Part print with two shaded views. Sizes in mm from the minimum x, y, z corner. A direction names the side the tool comes from. Coordinates: 2 decimals unless noted, no trailing zeros. Write each loop counter-clockwise with the first axis right and the second up, starting at its lowest first coordinate (ties: lowest second). Pieces come first, ordered by that corner, then holes. Notation, with made-up numbers: (86, 63.5) - (102, 63.5) arc R19 cw to (102, 90.5) - close; hole circle Ø8 at (-28.5, 16.5). An arc over 180 degrees is marked (long way). Answer in a Markdown table with one row per item. Add a question column.
Q1. Band-saw the part on A-A (y = 3.5). List the corners of the cut face in (x, z).
Q2. Band-saw the part on C-C (z = 1). List the corners of the cut face in (x, y).
Q3. Band-saw the part on B-B (x = 4). List the corners of the cut face in (y, z), and give its area (3 significant figures).
Q4. 3-axis set-ups, long thin cutter, end or side, ignore diameter. For the marked faces 1, 2 and 3: which of +Z, -Z, +X, -X, +Y, -Y reach the whole face in a straight line?
Q5. Drill centre lines: line 1 along Y through (x, z) = (37.5, 5.5); line 2 along Z through (x, y) = (4, 2.5); line 3 along X through (y, z) = (24, 5). Where is each one in solid material? Low to high. Write a range as from..to.
Q6. Band-saw the part on D-D (y = 29.5). List the corners of the cut face in (x, z), and give its area (3 significant figures).
Q7. Pin check, flat tips, straight feed: pin 1 (1.5 mm diameter, centred on y = 10, z = 5.5, fed in from -X); pin 2 (2 mm diameter, centred on y = 12.5, z = 5, fed in from +X); pin 3 (1.8 mm diameter, centred on x = 4, z = 3.75, fed in from -Y). Stop position of each tip, or through.
Q8. Two-plate mould, pull along Y, no slides. Class the marked faces 4, 5 and 6: +Y half, -Y half, draft (parallel to the pull), parting line (faces both ways), or undercut.
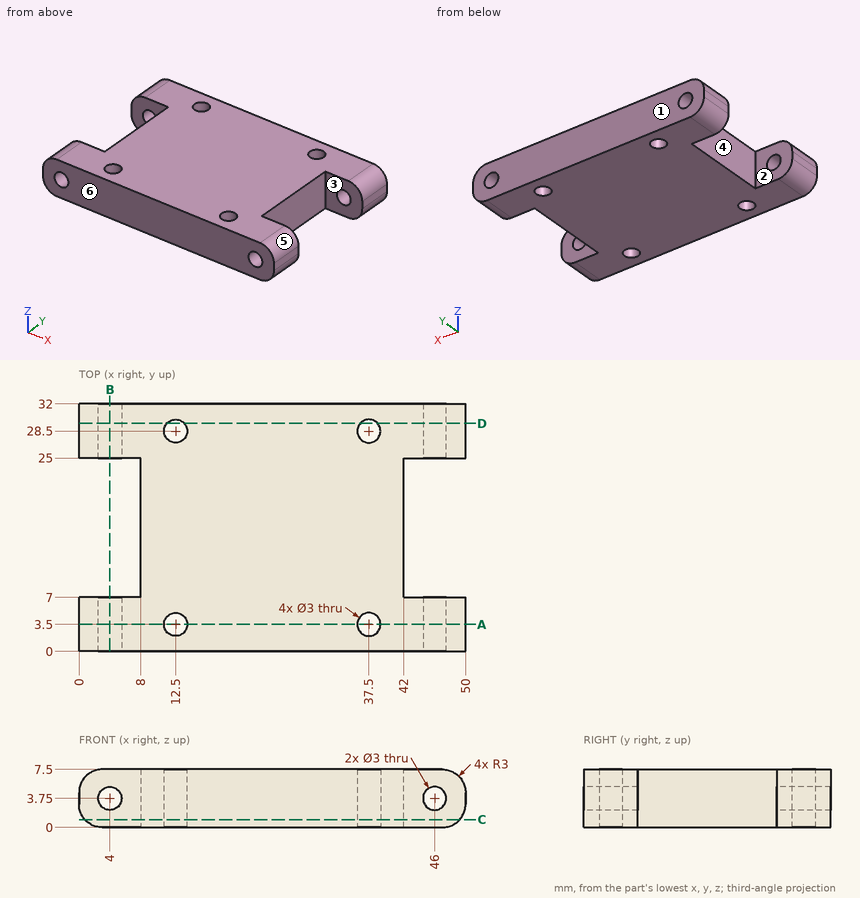
Checked values:
| question | item | result |
|---|---|---|
| 1 | outline | (0, 3) arc R3 ccw to (3, 0) - (11, 0) - (11, 7.5) - (3, 7.5) arc R3 ccw to (0, 4.5) - close; (14, 0) - (36, 0) - (36, 7.5) - (14, 7.5) - close; (39, 0) - (47, 0) arc R3 ccw to (50, 3) - (50, 4.5) arc R3 ccw to (47, 7.5) - (39, 7.5) - close; hole circle Ø3 at (4, 3.75); hole circle Ø3 at (46, 3.75) |
| 2 | outline | (0.76, 0) - (49.24, 0) - (49.24, 7) - (42, 7) - (42, 25) - (49.24, 25) - (49.24, 32) - (0.76, 32) - (0.76, 25) - (8, 25) - (8, 7) - (0.76, 7) - close; hole circle Ø3 at (12.5, 3.5); hole circle Ø3 at (12.5, 28.5); hole circle Ø3 at (37.5, 3.5); hole circle Ø3 at (37.5, 28.5) |
| 3 | outline | (0, 0) - (7, 0) - (7, 2.25) - (0, 2.25) - close; (0, 5.25) - (7, 5.25) - (7, 7.5) - (0, 7.5) - close; (25, 0) - (32, 0) - (32, 2.25) - (25, 2.25) - close; (25, 5.25) - (32, 5.25) - (32, 7.5) - (25, 7.5) - close |
| 3 | area | 63.0 mm² |
| 4 | face 1 | +Z, -Z, +X, -X, +Y |
| 4 | face 2 | +Z, -Z, -X |
| 4 | face 3 | +Z, -Z, +X |
| 5 | line 1 | y = 0..2, 5..27, 30..32 |
| 5 | line 2 | z = 0..2.25, 5.25..7.5 |
| 5 | line 3 | x = 8..42 |
| 6 | outline | (0, 3) arc R3 ccw to (3, 0) - (11.38, 0) - (11.38, 7.5) - (3, 7.5) arc R3 ccw to (0, 4.5) - close; (13.62, 0) - (36.38, 0) - (36.38, 7.5) - (13.62, 7.5) - close; (38.62, 0) - (47, 0) arc R3 ccw to (50, 3) - (50, 4.5) arc R3 ccw to (47, 7.5) - (38.62, 7.5) - close; hole circle Ø3 at (4, 3.75); hole circle Ø3 at (46, 3.75) |
| 6 | area | 320 mm² |
| 7 | pin 1 | stops at x = 8 |
| 7 | pin 2 | stops at x = 42 |
| 7 | pin 3 | passes through |
| 8 | face 4 | undercut |
| 8 | face 5 | draft |
| 8 | face 6 | -Y half |
